Read the model definition and answer for the solid it produces. Units are mm, in the model's axes. A direction names the side the tool comes from. Coordinates: 2 decimals unless noted, no trailing zeros. Loops run counter-clockwise (first coordinate to the right, second up) from the corner with the lowest first, then second, coordinate; pieces in that order, holes last. Notation, with made-up numbers: M 77.5,26.5 L 131.5,26.5 A31 cw 131.5,61.5 Z; hole C 2,-7.5 d4. An arc over 180 degrees is marked long. Put each result on its own line as item: value.
from build123d import *

# Parameters (mm, degrees)
SKETCH_1_R          = 6
EXTRUDE_1_DEPTH     = 10
SKETCH_2_R          = 5.7
SKETCH_3_R          = 6.9
CHAMFER_1_SIZE      = 0.5
CHAMFER_1_SIZE2     = 0.353553391
SKETCH_4_R          = 5
CUT_EXTRUDE_1_DEPTH = 2
SKETCH_5_R          = 4.5
EXTRUDE_2_DEPTH     = 2
CUT_EXTRUDE_2_DEPTH = 0.2
SKETCH_20_R         = 5
EXTRUDE_3_DEPTH     = 5.9
SKETCH_21_W         = 2
SKETCH_21_H         = 0.5
SKETCH_21_W_2       = 2.554126296
SKETCH_21_H_2       = 0.581017117
SKETCH_21_W_3       = 0.5
SKETCH_21_H_3       = 2
SKETCH_21_W_4       = 0.581017117
SKETCH_21_H_4       = 2.554126296
EXTRUDE_4_DEPTH     = 4.2


with BuildPart() as part:
    # 草图1 → 凸台-拉伸1 (new body)
    with BuildSketch(Plane(origin=(0, 0, 0), x_dir=(1, 0, 0), z_dir=(0, 1, 0))):
        with Locations(Location((0, 0, 0), (0, 0, 270))):
            Circle(SKETCH_1_R)
    extrude(amount=EXTRUDE_1_DEPTH)

    # 草图2 → 放样1 section 0
    with BuildSketch(Plane(origin=(0, 11.2, 0), x_dir=(1, 0, 0), z_dir=(0, 1, 0))):
        Circle(SKETCH_2_R)
    # 草图3 → 放样1 section 1
    with BuildSketch(Plane(origin=(0, 10, 0), x_dir=(1, 0, 0), z_dir=(0, 1, 0))):
        Circle(SKETCH_3_R)
    loft()

    # 倒角1
    chamfer_1_edges = [part.edges().sort_by_distance(p)[0] for p in [
        (-6.9, 10, 0),
    ]]
    chamfer_1_side = [part.faces().sort_by_distance(p)[0] for p in [
        (-6.704838528, 10, 0),
    ]]
    chamfer(chamfer_1_edges, length=CHAMFER_1_SIZE, length2=CHAMFER_1_SIZE2, reference=chamfer_1_side[0])

    # 草图4 → 切除-拉伸1 (cut)
    with BuildSketch(Plane(origin=(0, 11.2, 0), x_dir=(1, 0, 0), z_dir=(0, 1, 0))):
        with Locations(Location((0, 0, 0), (0, 0, 270))):
            Circle(SKETCH_4_R)
    extrude(amount=-CUT_EXTRUDE_1_DEPTH, mode=Mode.SUBTRACT)

    # 草图5 → 凸台-拉伸2 (add)
    with BuildSketch(Plane(origin=(0, 9.2, 0), x_dir=(1, 0, 0), z_dir=(0, 1, 0))):
        with Locations(Location((0, 0, 0), (0, 0, 270))):
            Circle(SKETCH_5_R)
    extrude(amount=EXTRUDE_2_DEPTH)

    # 草图6 → 切除-拉伸2 (cut)
    with BuildSketch(Plane(origin=(0, 11.2, 0), x_dir=(1, 0, 0), z_dir=(0, 1, 0))):
        with BuildLine():
            Line((-0.5, 0.5), (-0.5, 2))
            ThreePointArc((-0.5, 2), (0, 2.5), (0.5, 2))
            Line((0.5, 2), (0.5, 0.5))
            ThreePointArc((0.5, 0.5), (0, 0), (-0.5, 0.5))
        make_face()
        with BuildLine():
            ThreePointArc((-2.165063509, 1.25), (0, -2.5), (2.165063509, 1.25))
            ThreePointArc((2.165063509, 1.25), (1.482050808, 1.433012702), (1.299038106, 0.75))
            ThreePointArc((1.299038106, 0.75), (0, -1.5), (-1.299038106, 0.75))
            ThreePointArc((-1.299038106, 0.75), (-1.482050808, 1.433012702), (-2.165063509, 1.25))
        make_face()
    extrude(amount=-CUT_EXTRUDE_2_DEPTH, mode=Mode.SUBTRACT)

    # 草图20 → 凸台-拉伸3 (add)
    with BuildSketch(Plane.XZ):
        with Locations(Location((0, 0, 0), (0, 0, 90))):
            Circle(SKETCH_20_R)
    extrude(amount=EXTRUDE_3_DEPTH)

    # 草图21 → 凸台-拉伸4 (add)
    with BuildSketch(Plane.XZ.offset(5.9)):
        with Locations((0, 4.05)):
            Rectangle(SKETCH_21_W, SKETCH_21_H)
        with Locations((0, -4.090508558)):
            Rectangle(SKETCH_21_W_2, SKETCH_21_H_2)
        with Locations((4.05, 0)):
            Rectangle(SKETCH_21_W_3, SKETCH_21_H_3)
        with Locations((-4.090508558, 0)):
            Rectangle(SKETCH_21_W_4, SKETCH_21_H_4)
    extrude(amount=EXTRUDE_4_DEPTH)


solid = part.part
1) Find section B-B, the plane y = 1.5. Write down the section's boundary in (x, z).
Answer list:
outline: C 0,0 d12
2) Given pin 1 Ø0.6 at (y, z) = (-7, -4) entering from -X; pin 2 Ø1.5 at (x, y) = (0, 1.5) entering from -Z; pin 3 Ø3.5 at (x, z) = (-0.5, -1) entering from -Y, each flat-ended and moving along its own axis, determine where each tip first touches the part or whether it passes through.
Answer list:
pin 1: stops at x = -1.28
pin 2: stops at z = -6
pin 3: stops at y = -5.9
3) Determine the mould class of faces 5 (the flat face through (-4.381, -8, 0)), 6 (the cylindrical face through (1.352, 10.186, 4.292)), 7 (the flat face through (-1, 11.2, 0)), 8 (the flat face through (4.3, -8, 0)) for opening direction X: released by +X, released by -X, zero draft, split by the parting line, or undercut.
Answer list:
face 5: released by -X
face 6: undercut
face 7: zero draft
face 8: released by +X
4) Which of the six approach directions +Z, -Z, +X, -X, +Y, -Y give full straight-line access (tool end or side, diameter ignored) to faces 1 (the cylindrical face through (1.802, 4.93, 5.723)), 2 (the flat face through (0, -8, 4.3)), 3 (the flat face through (-3.8, -8, 0)), 4 (the flat face through (0, 11, 2))?
Answer list:
face 1: -Y
face 2: +Z, +X, -X, -Y
face 3: +Z, -Z, -Y
face 4: +Y
5) Find section A-A, the plane y = -7.5. Write down the section's boundary in (x, z).
Answer list:
outline: M -4.38,-1.28 L -3.8,-1.28 L -3.8,1.28 L -4.38,1.28 Z; M -1.28,-4.38 L 1.28,-4.38 L 1.28,-3.8 L -1.28,-3.8 Z; M -1,3.8 L 1,3.8 L 1,4.3 L -1,4.3 Z; M 3.8,-1 L 4.3,-1 L 4.3,1 L 3.8,1 Z
6) Find section C-C, the plane y = -4.5. Write down the section's boundary in (x, z).
Answer list:
outline: C 0,0 d10
7) Straight lines are drawn through the part: line 1 (X direction, y = 9.7, z = 0); line 2 (Y direction, x = -4.25, z = -1.75); line 3 (Y direction, x = -3, z = 1). For each, find the intervals that lie inside material, in ascending order. Write a range as [from, to].
Answer list:
line 1: x = [-6, -5], [-4.5, 4.5], [5, 6]
line 2: y = [-5.9, 9.2]
line 3: y = [-5.9, 11.2]
